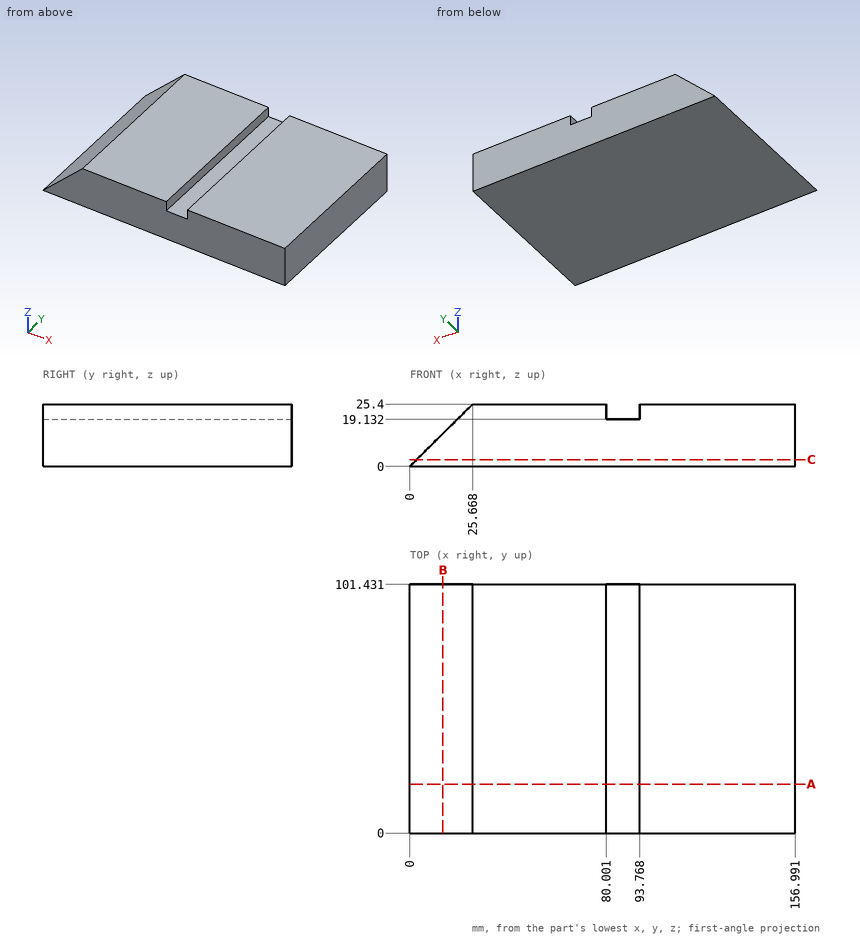
Could you check a few things on this drawing? It's one solid part, dimensions in mm from its lowest x, y, z. Give positions to 0.01 mm unless a question says otherwise; leave off trailing zeros. Write each loop counter-clockwise with the first axis right and the second up, starting at its lowest first coordinate (ties: lowest second). Pieces come first, ordered by that corner, then holes. Notation, with made-up numbers: (0.25, 46) -> (17.25, 46) arc R9 cw to (17.25, 50) -> close; hole circle Ø7 at (29.5, 13). An arc over 180 degrees is marked (long way). Answer as a JSON object with one key per item and string values.
Q1. Suppose I cut it at A-A on y = 20. Write out the boundary of the cut face in (x, z).
Taken from the geometry:
{"outline": "(0, 0) -> (156.99, 0) -> (156.99, 25.4) -> (93.77, 25.4) -> (93.77, 19.13) -> (80, 19.13) -> (80, 25.4) -> (25.67, 25.4) -> close"}
Q2. Please list where these lines run through material, in increasing order: L1, parallel to Z at x = 83, y = 57; L2, parallel to X at y = 21, z = 24.5; L3, parallel to X at y = 72, z = 4.
Taken from the geometry:
{"L1": "z = 0 to 19.13", "L2": "x = 24.76 to 80, 93.77 to 156.99", "L3": "x = 4.04 to 156.99"}
Q3. Suppose I cut it at B-B on x = 13.5. Write out the boundary of the cut face in (y, z), then the cut area to 4 significant figures.
Taken from the geometry:
{"outline": "(0, 0) -> (101.43, 0) -> (101.43, 13.36) -> (0, 13.36) -> close", "area": "1,355 mm²"}
Q4. Suppose I cut it at C-C on z = 2.75. Write out the boundary of the cut face in (x, y), then the cut area to 3 significant figures.
Taken from the geometry:
{"outline": "(2.78, 0) -> (156.99, 0) -> (156.99, 101.43) -> (2.78, 101.43) -> close", "area": "15,600 mm²"}
Q5. Will these pins go through, and if not, where does the flat tip stop? pin 1 Ø7 at (x, y) = (84.5, 27.5) entering from +Z; pin 2 Ø3 at (y, z) = (70, 22.5) entering from -X.
Taken from the geometry:
{"pin 1": "stops at z = 19.13", "pin 2": "stops at x = 21.22"}
